Could you check a few things on this model? Use its own coordinates, in mm. Give positions to 0.01 mm unless a question says otherwise; leave off trailing zeros. Order: outer loops, then holes, each group sorted by start corner. A loop starts at its lowest first (then second) coordinate and runs counter-clockwise, first axis right, second up. Notation, with made-up numbers: M 54.25,1 L 112.25,1 A18 cw 112.25,27 Z; hole C -16.75,86.25 d2. An arc over 180 degrees is marked long. Answer in a Markdown table with one row per item. Add a question column.
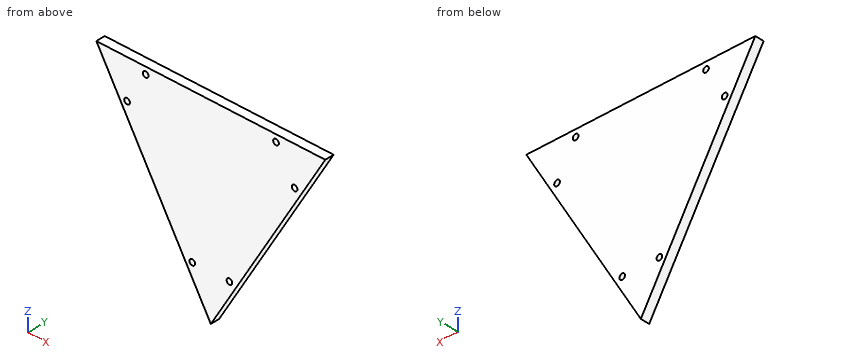
```python
from build123d import *

# Parameters (mm, degrees)
SALIENTE_EXTRUIR2_DEPTH = 8
CROQUIS3_R              = 2.5
CORTAR_EXTRUIR1_DEPTH   = 31


with BuildPart() as part:
    # Croquis1 → Saliente-Extruir2 (new body)
    with BuildSketch(Plane(origin=(0, 0, 0), x_dir=(1, 0, 0), z_dir=(0, 1, 0))):
        Polygon((101.602540378, 0), (0, 175.908017141), (-101.602540378, 0), align=None)
    extrude(amount=SALIENTE_EXTRUIR2_DEPTH)

    # Croquis3 → Cortar-Extruir1 (cut)
    with BuildSketch(Plane(origin=(0, 8, 0), x_dir=(1, 0, 0), z_dir=(0, 1, 0))):
        with Locations(Location((-16.5, 135, 0), (0, 0, 270))):
            Circle(CROQUIS3_R)
        with Locations(Location((16.5, 135, 0), (0, 0, 270))):
            Circle(CROQUIS3_R)
        with Locations(Location((-57.862159322, 6.200961894, 0), (0, 0, 270))):
            Circle(CROQUIS3_R)
        with Locations(Location((-74.362159322, 34.779800219, 0), (0, 0, 270))):
            Circle(CROQUIS3_R)
        with Locations(Location((57.862159322, 6.200961894, 0), (0, 0, 270))):
            Circle(CROQUIS3_R)
        with Locations(Location((74.362159322, 34.779800219, 0), (0, 0, 270))):
            Circle(CROQUIS3_R)
    extrude(amount=-CORTAR_EXTRUIR1_DEPTH, mode=Mode.SUBTRACT)


solid = part.part
```
1. Suppose I cut it at B-B on y = 2. List the corners of the cut face in (x, z) for me.
2. Will these pins go through, and if not, where does the flat tip stop? P1, Ø4, axis at y = 6.5, z = -141.5, coming from the +X side; P2, Ø4, axis at y = 5, z = -123, coming from the -X side; P3, Ø3, axis at x = 57.86, z = -6.2, coming from the -Y side; P4, Ø1.5, axis at y = 5, z = -128, coming from the -X side.
3. Suppose I cut it at A-A on z = -135. List the corners of the cut face in (x, y) for me.
4. Suppose I cut it at C-C on x = -16.5. List the corners of the cut face in (y, z) for me, plus the area to 3 significant figures.
5. If I drill on line 1 along X through (y, z) = (4.5, -135); line 2 along X through (y, z) = (7.25, -133); line 3 along Z through (x, y) = (-18, 5.75), over which ranges is the centre line in solid material (lowest first)? Write a range as [from, to].
6. Suppose I cut it at D-D on x = -84.5. List the corners of the cut face in (y, z) for me.
Findings below:
| question | item | result |
|---|---|---|
| 1 | outline | M -101.6,0 L 0,-175.91 L 101.6,0 Z; hole C -74.36,-34.78 d5; hole C -57.86,-6.2 d5; hole C -16.5,-135 d5; hole C 16.5,-135 d5; hole C 57.86,-6.2 d5; hole C 74.36,-34.78 d5 |
| 2 | P1 | x = 21.03 |
| 2 | P2 | x = -31.71 |
| 2 | P3 | through |
| 2 | P4 | x = -28.1 |
| 3 | outline | M -23.63,0 L -19,0 L -19,8 L -23.63,8 Z; M -14,0 L 14,0 L 14,8 L -14,8 Z; M 19,0 L 23.63,0 L 23.63,8 L 19,8 Z |
| 4 | outline | M 0,-147.34 L 8,-147.34 L 8,-137.5 L 0,-137.5 Z; M 0,-132.5 L 8,-132.5 L 8,0 L 0,0 Z |
| 4 | area | 1,140 mm2 |
| 5 | line 1 | [-23.63, -19], [-14, 14], [19, 23.63] |
| 5 | line 2 | [-24.78, -18], [-15, 15], [18, 24.78] |
| 5 | line 3 | [-144.74, -137], [-133, 0] |
| 6 | outline | M 0,-29.61 L 8,-29.61 L 8,0 L 0,0 Z |
